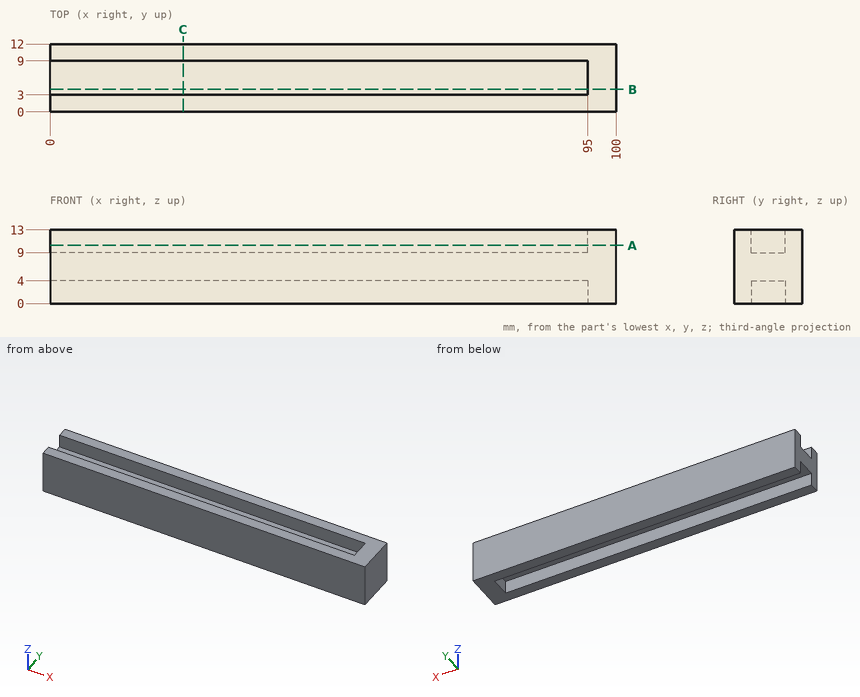
Geometry check sheet. Reference: drawing and pictorial views, mm from the part's lowest x, y, z. Coordinates: 2 decimals unless noted, no trailing zeros. Write each loop counter-clockwise with the first axis right and the second up, starting at its lowest first coordinate (ties: lowest second). Pieces come first, ordered by that corner, then holes. Notation, with made-up numbers: M 71.5,-30 L 103.5,-30 A18 cw 103.5,-22 Z; hole C 35.5,79 d4. An arc over 180 degrees is marked long. One line per question, with ' | ' between items.
1) Sectioned sample at B-B on y = 4. Record the cut outline in (x, z), then the cut area to 3 significant figures.
Solutions:
outline: M 0,4 L 95,4 L 95,0 L 100,0 L 100,13 L 95,13 L 95,9 L 0,9 Z | area: 540 mm^2
2) Material ranges on L1, parallel to Y at x = 76, z = 2.75; L2, parallel to X at y = 5.5, z = 10.75; L3, parallel to Z at x = 20, y = 3.25, recorded low to high.
Solutions:
L1: 0 to 3, 9 to 12 | L2: 95 to 100 | L3: 4 to 9
3) Depth check by flat-ended pin: pin 1 Ø5 at (x, y) = (57, 6) entering from +Z; pin 2 Ø3 at (x, y) = (45, 5.5) entering from -Z. Enter the tip coordinate at first touch or a pass-through.
Solutions:
pin 1: z = 9 | pin 2: z = 4
4) Sectioned sample at A-A on z = 10.25. Record the cut outline in (x, y).
Solutions:
outline: M 0,0 L 100,0 L 100,12 L 0,12 L 0,9 L 95,9 L 95,3 L 0,3 Z
5) Sectioned sample at C-C on x = 23.5. Record the cut outline in (y, z), then the cut area to 3 significant figures.
Solutions:
outline: M 0,0 L 3,0 L 3,4 L 9,4 L 9,0 L 12,0 L 12,13 L 9,13 L 9,9 L 3,9 L 3,13 L 0,13 Z | area: 108 mm^2
